```python
from build123d import *

# Parameters (mm, degrees)
SKETCH1_W           = 203.2
SKETCH1_H           = 38.1
SKETCH1_R           = 12.7
BOSS_EXTRUDE1_DEPTH = 7.62
FILLET1_R           = 19.05


with BuildPart() as part:
    # Sketch1 → Boss-Extrude1 (new body)
    with BuildSketch(Plane.XY):
        Rectangle(SKETCH1_W, SKETCH1_H)
        with Locations(Location((-81.28, 0, 0), (0, 0, 180))):
            Circle(SKETCH1_R, mode=Mode.SUBTRACT)
        with Locations(Location((82.317778023, 0, 0), (0, 0, 180))):
            Circle(SKETCH1_R, mode=Mode.SUBTRACT)
        with BuildLine():
            Line((-52.511607643, 8.682983434), (49.088392357, 8.682983434))
            ThreePointArc((49.088392357, 8.682983434), (57.771375791, 0), (49.088392357, -8.682983434))
            Line((49.088392357, -8.682983434), (-52.511607643, -8.682983434))
            ThreePointArc((-52.511607643, -8.682983434), (-61.194591077, 0), (-52.511607643, 8.682983434))
        make_face(mode=Mode.SUBTRACT)
    extrude(amount=BOSS_EXTRUDE1_DEPTH)

    # Fillet1
    fillet1_edges = [part.edges().sort_by_distance(p)[0] for p in [
        (101.6, -19.05, 3.81),
        (101.6, 19.05, 3.81),
        (-101.6, -19.05, 3.81),
        (-101.6, 19.05, 3.81),
    ]]
    fillet(fillet1_edges, radius=FILLET1_R - 0.0001)  # a hair under: the kernel refuses the full size


solid = part.part
```
Source: CAD feature listing. Evaluate the final solid. Frame: model axes, mm. A direction names the side the tool comes from. Round coordinates to 2 decimals unless told otherwise and drop trailing zeros. Loops run counter-clockwise (first coordinate to the right, second up) from the corner with the lowest first, then second, coordinate; pieces in that order, holes last. Notation, with made-up numbers: M -40,72 L -20,72 A28 cw -20,92 Z; hole C -5.75,3.5 d11. An arc over 180 degrees is marked long. Use a Markdown table: item, result. Add a question column.
1. Cut plane C-C, the plane x = 80. Output: boundary loops of the cut face in (y, z).
2. Set-up query: faces 1 (the flat face through (-1, -8.683, 4)), 2 (the flat face through (-1, -19.05, 4)). Return all of +Z, -Z, +X, -X, +Y, -Y with unobstructed straight access to the full face (end or side cutting, diameter ignored); none if empty.
3. Cut plane B-B, the plane z = 5. State how many separate pieces and enclosed holes the cut face has, and give its area (3 significant figures).
4. Pull-direction query (X, two-part tool) for faces 3 (the cylindrical face through (-96.17, -13.32, 3.86)), 4 (the cylindrical face through (-68.592, -0.558, 3.757)), 5 (the flat face through (-2, 8.683, 4)), 6 (the flat face through (-1, 9, 0)); classes: +X half, -X half, draft (parallel to the pull), parting line (faces both ways), or undercut.
5. Contact query for flat-ended pins moving along their axis: pin 1 (4 mm diameter, centred on y = 2.5, z = 1.5, fed in from -X); pin 2 (4 mm diameter, centred on y = -4, z = 5.5, fed in from -X). Output: stop coordinate, or through.
6. Ray query, line 1 along X through (y, z) = (5, 5); line 2 along Y through (x, z) = (-81.28, 6); line 3 along Y through (x, z) = (-1, 4.25). Return the intervals inside material, ascending. Write a range as [from, to].
7. Cut plane A-A, the plane x = -47. Output: boundary loops of the cut face in (y, z), and give its area (3 significant figures).
Solution:
| question | item | result |
|---|---|---|
| 1 | outline | M -19.05,0 L -12.49,0 L -12.49,7.62 L -19.05,7.62 Z; M 12.49,0 L 19.05,0 L 19.05,7.62 L 12.49,7.62 Z |
| 2 | face 1 | +Z, -Z |
| 2 | face 2 | +Z, -Z, +X, -X, -Y |
| 3 | separate pieces | 1 |
| 3 | enclosed holes | 3 |
| 3 | area | 4,420 mm2 |
| 4 | face 3 | -X half |
| 4 | face 4 | undercut |
| 4 | face 5 | undercut |
| 4 | face 6 | draft |
| 5 | pin 1 | stops at x = -101.59 |
| 5 | pin 2 | stops at x = -101.49 |
| 6 | line 1 | x = [-100.93, -92.95], [-69.61, -59.61], [56.19, 70.64], [93.99, 100.93] |
| 6 | line 2 | y = [-19.05, -12.7], [12.7, 19.05] |
| 6 | line 3 | y = [-19.05, -8.68], [8.68, 19.05] |
| 7 | outline | M -19.05,0 L -8.68,0 L -8.68,7.62 L -19.05,7.62 Z; M 8.68,0 L 19.05,0 L 19.05,7.62 L 8.68,7.62 Z |
| 7 | area | 158 mm2 |
